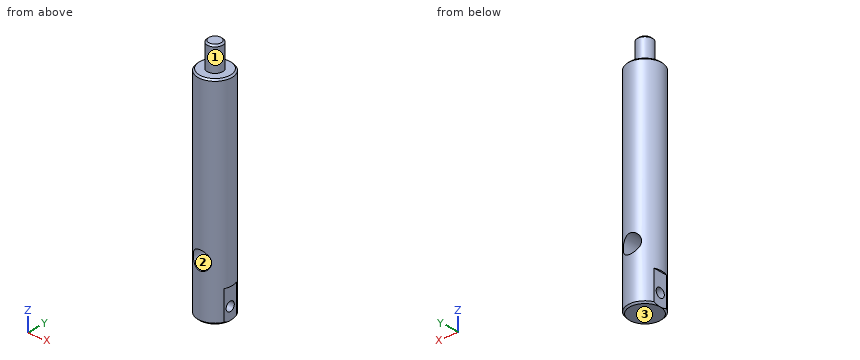
```python
from build123d import *

# Parameters (mm, degrees)
SKETCH_1_R          = 5.5
EXTRUDE_1_DEPTH     = 69.5
CHAMFER_1_SIZE      = 0.5
SKETCH_2_R          = 2.5
EXTRUDE_2_DEPTH     = 8
CHAMFER_2_SIZE      = 0.5
SKETCH_5_R          = 1.5
CUT_EXTRUDE_3_DEPTH = 7.5
SKETCH_6_R          = 3
CUT_EXTRUDE_4_DEPTH = 7.5
SKETCH_7_W          = 2
SKETCH_7_H          = 10
CUT_EXTRUDE_5_DEPTH = 10


with BuildPart() as part:
    # 草图1 → 拉伸1 (new body)
    with BuildSketch(Plane.XY):
        Circle(SKETCH_1_R)
    extrude(amount=EXTRUDE_1_DEPTH)

    # 倒角1
    chamfer_1_edges = [part.edges().sort_by_distance(p)[0] for p in [
        (-5.5, 0, 0),
        (-5.5, 0, 69.5),
    ]]
    chamfer(chamfer_1_edges, length=CHAMFER_1_SIZE)

    # 草图2 → 拉伸2 (add)
    with BuildSketch(Plane.XY.offset(69.5)):
        Circle(SKETCH_2_R)
    extrude(amount=EXTRUDE_2_DEPTH)

    # 倒角2
    chamfer_2_edges = [part.edges().sort_by_distance(p)[0] for p in [
        (-2.5, 0, 77.5),
    ]]
    chamfer(chamfer_2_edges, length=CHAMFER_2_SIZE)

    # 草图5 → 拉伸3 (cut, symmetric)
    with BuildSketch(Plane(origin=(0, 0, 0), x_dir=(0, 0, -1), z_dir=(1, 0, 0))):
        with Locations(Location((-4, 0, 0), (0, 0, 180))):
            Circle(SKETCH_5_R)
    extrude(amount=CUT_EXTRUDE_3_DEPTH, both=True, mode=Mode.SUBTRACT)

    # 草图6 → 拉伸4 (cut, symmetric)
    with BuildSketch(Plane(origin=(0, 0, 0), x_dir=(1, 0, 0), z_dir=(0, 1, 0))):
        with Locations(Location((0, -17.5, 0), (0, 0, 270))):
            Circle(SKETCH_6_R)
    extrude(amount=CUT_EXTRUDE_4_DEPTH, both=True, mode=Mode.SUBTRACT)

    # 草图7 → 拉伸5 (cut)
    with BuildSketch(Plane.XY):
        with Locations((6, 0)):
            Rectangle(SKETCH_7_W, SKETCH_7_H)
    cut_extrude_5 = extrude(amount=CUT_EXTRUDE_5_DEPTH, mode=Mode.SUBTRACT)

    # 镜向1: 拉伸5 across plane
    add(cut_extrude_5.mirror(Plane(origin=(0, 0, 0), x_dir=(0, 0, 1), z_dir=(1, 0, 0))), mode=Mode.SUBTRACT)


solid = part.part
```
Geometry check sheet. Reference: the model listing, model coordinates, mm. Face numbers are marked on the shaded views. Give positions to 0.01 mm unless a question says otherwise; leave off trailing zeros. Loops run counter-clockwise (first coordinate to the right, second up) from the corner with the lowest first, then second, coordinate; pieces in that order, holes last. Notation, with made-up numbers: M 72.5,1 L 116.5,1 A31 cw 116.5,31 Z; hole C 32,8.5 d4. An arc over 180 degrees is marked long. Write item = value, one per line. Start each with the question number.
1. Section check B-B, the plane z = 4. Enter the section's corners in (x, y).
2. Section check C-C, the plane z = 31.5. Enter the section's corners in (x, y), plus the area to 3 significant figures.
3. Section check D-D, the plane z = 17.5. Enter the section's corners in (x, y).
4. Go/stop test with flat-tipped pins: P1, Ø2, axis at x = 2.5, z = 50, coming from the -Y side; P2, Ø2, axis at y = -1.5, z = 46, coming from the -X side; P3, Ø1, axis at y = 2, z = 36, coming from the -X side. Record where each tip stops, or that it passes through.
5. Section check A-A, the plane x = 0. Enter the section's corners in (y, z), plus the area to 3 significant figures.
6. Draft check along Z on the marked faces 1, 2 and 3. Enter one of: +Z half, -Z half, draft (parallel to the pull), parting line (faces both ways), or undercut.
7. Thickness scan on probe 1 along X at (y, z) = (-1, 5.5); probe 2 along X at (y, z) = (2.5, 17.5); probe 3 along Z at (x, y) = (-1.5, -3). Record the ranges inside material, lowest first.
Values follow:
q1.outline = M -5,-2.29 A5.5 ccw 5,-2.29 L 5,-1.5 L -5,-1.5 Z; M -5,1.5 L 5,1.5 L 5,2.29 A5.5 ccw -5,2.29 Z
q2.outline = C 0,0 d11
q2.area = 95.0 mm^2
q3.outline = M -3,-4.61 L -3,4.61 A5.5 ccw Z; M 3,-4.61 A5.5 ccw 3,4.61 Z
q4.P1 = -5.29
q4.P2 = -5.48
q4.P3 = -5.29
q5.outline = M -5.5,0.5 L -5,0 L 5,0 L 5.5,0.5 L 5.5,14.5 L -5.5,14.5 Z; M -5.5,20.5 L 5.5,20.5 L 5.5,69 L 5,69.5 L 2.5,69.5 L 2.5,77 L 2,77.5 L -2,77.5 L -2.5,77 L -2.5,69.5 L -5,69.5 L -5.5,69 Z; hole C 0,4 d3
q5.area = 731 mm^2
q6.face_1 = draft
q6.face_2 = undercut
q6.face_3 = -Z half
q7.probe_1 = -5 to 5
q7.probe_2 = -4.9 to -3, 3 to 4.9
q7.probe_3 = 0 to 14.9, 20.1 to 69.5
